Autodesk Inventor part; units mm, degrees
ref_plane "YZ Plane" through (0, 0, 0) normal (1, 0, 0) x (0, 1, 0)
ref_plane "XZ Plane" through (0, 0, 0) normal (0, 1, 0) x (-1, 0, 0)
ref_plane "XY Plane" through (0, 0, 0) normal (0, 0, 1) x (1, 0, 0)
ref_plane "Work Plane1" through (0, 0, 0) normal (0, 0, 1) x (1, 0, 0)
sketch "Sketch1" plane through (0, 0, 0) normal (0, 0, 1) x (1, 0, 0)
  line L0 (0, 0) -> (5.55, 0)
  line L1 (6.05, -7.8) -> (0, -7.8)
  line L2 (0, -7.8) -> (0, 0)
  line L3 (5.55, 0) -> (6.05, -0.5)
  arc A0 (6.05, -3.6294) -> (5.8482, -3.4873) centre (5.8013, -3.7683) ccw
  arc A1 (5.5514, -3.0941) -> (5.8482, -3.4873) centre (6.6343, -2.5853) ccw
  arc A2 (5.5514, -3.0941) -> (5.425, -2.9829) centre (5.3332, -3.2146) ccw
  line L4 (5.425, -2.9829) -> (4.928, -2.9441)
  arc A3 (4.7, -2.7255) -> (4.928, -2.9441) centre (4.9475, -2.6956) ccw
  arc A4 (4.9275, -2.0261) -> (4.7, -2.2744) centre (4.9493, -2.2744) ccw
  arc A5 (5.293, -1.9942) -> (5.5514, -1.8412) centre (5.3208, -1.7464) ccw
  arc A6 (5.8954, -1.3233) -> (5.5514, -1.8412) centre (6.7024, -2.2326) ccw
  arc A7 (5.8954, -1.3233) -> (6.05, -1.1) centre (5.8008, -1.0927) ccw
  line L5 (5.293, -1.9942) -> (4.9275, -2.0261)
  line L6 (4.7, -2.7255) -> (4.7, -2.2744)
  line L7 (6.05, -0.5) -> (6.05, -1.1)
  line L8 (6.05, -3.6294) -> (6.05, -7.8)
  point P0 (6.05, 0)
  dimension "d0" = 0.5
  dimension "d1" = 0.5
  dimension "d17" = 6.05
  dimension "d18" = 7.8
  dimension "d20" = 2.6756
  dimension "d21" = 0.5
  dimension "d22" = 1.1
  dimension "d23" = 4.7
  dimension "d24" = 0.2275
  dimension "d25" = 0.228
  dimension "d26" = 0
  dimension "d27" = 0.2483
  dimension "d28" = 0.2186
extrude "Extrusion1" add sketch "Sketch1" along normal blind 50
mirror "Mirror1" about plane through (0, 0, 0) normal (-1, 0, 0) of "Extrusion1"
sketch "Sketch2" plane through (5.55, 0, 50) normal (0, 1, 0) x (1, 0, 0)
  line L0 (-11.1, 50) -> (0, 50)
  line L1 (-11.1, 50) -> (-11.1, 0)
  line L2 (0, 0) -> (-11.1, 0)
  line L3 (0, 50) -> (0, 0)
  point P0 (-5.55, 50)
  point P1 (-5.45, 45.5983)
hole "Hole1" at (0.1, 0, 4.4017) direction (0, -1, 0) diameter 3.5 end through all counterbore diameter 7 counterbore depth 3.5
pattern_linear "Rectangular Pattern1" count 5 spacing 12.5 along (0, 0, 1) of "Hole1"
ref_plane "Work Plane2" through (0, -7.8, 0) normal (1, 0, 0) x (0, 0, -1)
ref_plane "Arbeitsebene3" through (0, 0, 25) normal (0, 0, 1) x (1, 0, 0)
pattern_linear "Rechteckige Anordnung2" count 3 spacing 50 along (0, 0, 1) of "Extrusion1", "Mirror1", "Hole1", "Rectangular Pattern1"
ref_plane "Arbeitsebene4" through (0, 0, 75) normal (0, 0, -1) x (-1, 0, 0)
ref_plane "Arbeitsebene5" through (0, -7.8, 0) normal (-1, 0, 0) x (0, 0, 1)
properties part number "30_Cube_Z_Focus_MGN_NEMA_rail"
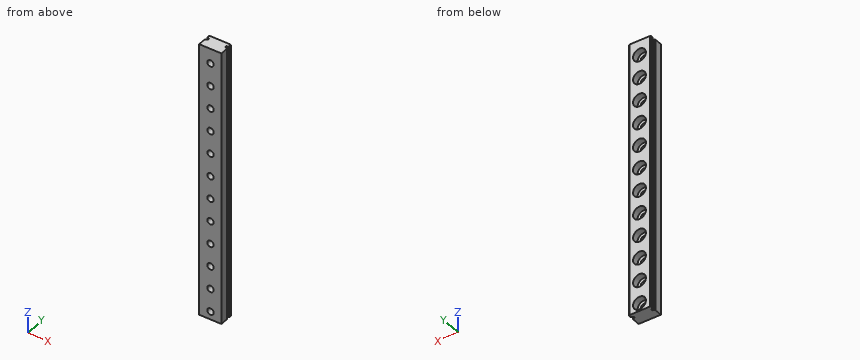
Input: part model. Units: mm. Frame: model coordinates. Coordinates: 2 decimals unless noted, no trailing zeros.
1) Material intervals for line 1 along Y through (x, z) = (1, 127.5); line 2 along X through (y, z) = (-2.75, 70); line 3 along X through (y, z) = (-4.25, 104.5), sorted ascending.
2) Pin query (flat end, axial travel): pin 1 Ø4.5 at (x, z) = (0.1, 41.9) entering from +Y. Return the tip coordinate at first contact, or that it passes through.
3) Section B-B on x = 0.1. State how many separate pieces and enclosed holes the cut face has, and give its area (3 significant figures).
Check result:
1. line 1: y = -7.8 to -3.5
1. line 2: x = -4.7 to -1.53, 1.73 to 4.7
1. line 3: x = -6.05 to -1.65, 1.85 to 6.05
2. pin 1: stops at y = -3.5
3. separate pieces: 13
3. enclosed holes: 0
3. area: 695 mm2
